Work out the finished part from the listing and answer in its coordinate system (mm). A direction names the side the tool comes from. Give positions to 0.01 mm unless a question says otherwise; leave off trailing zeros. Loops run counter-clockwise (first coordinate to the right, second up) from the corner with the lowest first, then second, coordinate; pieces in that order, holes last. Notation, with made-up numbers: M 0.5,-7.75 L 50.5,-7.75 A14 cw 50.5,9.25 Z; hole C 8.5,73 d1. An arc over 180 degrees is marked long. Answer as a JSON object with one key per item and string values. Group by question number.
```python
from build123d import *

# Parameters (mm, degrees)
SKETCH1_R           = 31.75
SKETCH1_R_2         = 2.794
BOSS_EXTRUDE3_DEPTH = 6.35
FILLET1_R           = 3.81


with BuildPart() as part:
    # Sketch1 → Boss-Extrude3 (new body)
    with BuildSketch(Plane.XY):
        Circle(SKETCH1_R)
        with BuildLine():
            Line((-18.730057548, -15.213212818), (0, -4.399409051))
            Line((0, -4.399409051), (18.730057548, -15.213212818))
            ThreePointArc((18.730057548, -15.213212818), (0, -24.13), (-18.730057548, -15.213212818))
        make_face(mode=Mode.SUBTRACT)
        with BuildLine():
            Line((-3.81, 23.82731206), (-3.81, 2.199704526))
            Line((-3.81, 2.199704526), (-22.540057548, -8.614099242))
            ThreePointArc((-22.540057548, -8.614099242), (-20.897192993, 12.065), (-3.81, 23.82731206))
        make_face(mode=Mode.SUBTRACT)
        Circle(SKETCH1_R_2, mode=Mode.SUBTRACT)
        with BuildLine():
            Line((22.540057548, -8.614099242), (3.81, 2.199704526))
            Line((3.81, 2.199704526), (3.81, 23.82731206))
            ThreePointArc((3.81, 23.82731206), (20.897192993, 12.065), (22.540057548, -8.614099242))
        make_face(mode=Mode.SUBTRACT)
    extrude(amount=BOSS_EXTRUDE3_DEPTH)

    # Fillet1
    fillet1_edges = [part.edges().sort_by_distance(p)[0] for p in [
        (18.730057548, -15.213212818, 3.175),
        (0, -4.399409051, 3.175),
        (-18.730057548, -15.213212818, 3.175),
        (3.81, 23.82731206, 3.175),
        (3.81, 2.199704526, 3.175),
        (22.540057548, -8.614099242, 3.175),
        (-22.540057548, -8.614099242, 3.175),
        (-3.81, 2.199704526, 3.175),
        (-3.81, 23.82731206, 3.175),
    ]]
    fillet(fillet1_edges, radius=FILLET1_R)


solid = part.part
```
Item 1: A cutting plane is placed at D-D (y = -18). Determine the outline of the cut face in (x, z), and give its area (3 significant figures).
Item 2: Given pin 1 Ø1.5 at (y, z) = (-8.5, 2.5) entering from -X; pin 2 Ø1.9 at (y, z) = (15, 2) entering from -X; pin 3 Ø1.5 at (x, z) = (-11, 3.5) entering from -Y, each flat-ended and moving along its own axis, determine where each tip first touches the part or whether it passes through.
Item 3: A cutting plane is placed at B-B (x = 0). Determine the outline of the cut face in (y, z), and give its area (3 significant figures).
Item 4: A cutting plane is placed at A-A (y = 0). Determine the outline of the cut face in (x, z).
Item 5: For a pull along Y with two mould halves and no side action, classify faces 3 (the cylindrical face through (-6.883, -30.995, 3.131)), 4 (the flat face through (7, 0, 6.35)), 5 (the cylindrical face through (-16.307, -15.805, 3.219)) as pulls with the +Y half, pulls with the -Y half, needs draft (parallel to the pull), parting line crosses it, or undercut.
Item 6: A cutting plane is placed at C-C (z = 1). Determine the outline of the cut face in (x, y) (3 decimals), and give its area (3 significant figures).
Item 7: A tool of negligible diameter and unlimited length cuts with its end or side. For faces 1 (the flat face through (7, 0, 0)), 2 (the flat face through (12.054, -2.56, 3.131)), from which of +Z, -Z, +X, -X, +Y, -Y can it reach the whole face along a straight path? Write none if from no direction.
Item 8: Find the intervals of material crossed by probe 1 along Y at (x, z) = (0, 3.5); probe 2 along X at (y, z) = (0.5, 6.25); probe 3 along X at (y, z) = (12.5, 3.5), in increasing order. Write a range as [from, to].
The answers:
{
 "1": {"outline": "M -26.15,0 L -15.76,0 L -15.76,6.35 L -26.15,6.35 Z; M 15.76,0 L 26.15,0 L 26.15,6.35 L 15.76,6.35 Z", "area": "132 mm^2"},
 "2": {"pin 1": "stops at x = -30.79", "pin 2": "stops at x = -28.47", "pin 3": "stops at y = -30.05"},
 "3": {"outline": "M -31.75,0 L -24.13,0 L -24.13,6.35 L -31.75,6.35 Z; M -4.99,0 L -2.79,0 L -2.79,6.35 L -4.99,6.35 Z; M 2.79,0 L 31.75,0 L 31.75,6.35 L 2.79,6.35 Z", "area": "246 mm^2"},
 "4": {"outline": "M -31.75,0 L -24.13,0 L -24.13,6.35 L -31.75,6.35 Z; M -7.62,0 L -2.79,0 L -2.79,6.35 L -7.62,6.35 Z; M 2.79,0 L 7.62,0 L 7.62,6.35 L 2.79,6.35 Z; M 24.13,0 L 31.75,0 L 31.75,6.35 L 24.13,6.35 Z"},
 "5": {"face 3": "parting line crosses it", "face 4": "needs draft", "face 5": "undercut"},
 "6": {"outline": "C 0,0 d63.5; hole M -23.897,-3.348 A3.81 ccw -18.218,-6.119 L -5.715,1.1 A3.81 ccw -3.81,4.399 L -3.81,18.837 A3.81 ccw -9.049,22.369 A24.13 ccw Z; hole M -14.848,-19.021 A24.13 ccw 14.848,-19.021 A3.81 ccw 14.408,-12.718 L 1.905,-5.499 A3.81 ccw -1.905,-5.499 L -14.408,-12.718 A3.81 ccw Z; hole C 0,0 d5.588; hole M 3.81,4.399 A3.81 ccw 5.715,1.1 L 18.218,-6.119 A3.81 ccw 23.897,-3.348 A24.13 ccw 9.049,22.369 A3.81 ccw 3.81,18.837 Z", "area": "1,880 mm^2"},
 "7": {"face 1": "-Z, +X, -X, +Y, -Y", "face 2": "+Z, -Z"},
 "8": {"probe 1": "y = [-31.75, -24.13], [-4.99, -2.79], [2.79, 31.75]", "probe 2": "x = [-31.75, -24.12], [-6.75, -2.75], [2.75, 6.75], [24.12, 31.75]", "probe 3": "x = [-29.19, -20.64], [-3.81, 3.81], [20.64, 29.19]"}
}
